Could you check a few things on this model? Use its own coordinates, in mm. A direction names the side the tool comes from. Coordinates: 2 decimals unless noted, no trailing zeros. Order: outer loops, then holes, each group sorted by start corner. A loop starts at its lowest first (then second) coordinate and runs counter-clockwise, first axis right, second up.
```python
from build123d import *

# Parameters (mm, degrees)
SKETCH1_W               = 200
SKETCH1_H               = 180
BOSS_EXTRUDE1_DEPTH     = 90
CUT_EXTRUDE1_DEPTH      = 1
CUT_EXTRUDE1_DEPTH_BACK = 181
CUT_EXTRUDE2_DEPTH      = 201
SHELL1_T                = -1.5
SKETCH6_R               = 2.25
HINGE_HOLES_DEPTH       = 2.5
CUT_EXTRUDE4_DEPTH      = 50


with BuildPart() as part:
    # Sketch1 → Boss-Extrude1 (new body)
    with BuildSketch(Plane(origin=(0, 0, 0), x_dir=(1, 0, 0), z_dir=(0, 1, 0))):
        with Locations((100, 90)):
            Rectangle(SKETCH1_W, SKETCH1_H)
    extrude(amount=BOSS_EXTRUDE1_DEPTH)

    # Sketch4 → Cut-Extrude1 (cut, two sides)
    with BuildSketch(Plane.XY) as cut_extrude1_sk:
        Polygon((0, 85), (30.937469913, 0), (0, 0), align=None)
        Polygon((200, 85), (200, 0), (169.062530087, 0), align=None)
    extrude(amount=CUT_EXTRUDE1_DEPTH, mode=Mode.SUBTRACT)
    extrude(cut_extrude1_sk.sketch, amount=-CUT_EXTRUDE1_DEPTH_BACK, mode=Mode.SUBTRACT)

    # Sketch5 → Cut-Extrude2 (cut, through all)
    with BuildSketch(Plane.ZY):
        Polygon((-180, 85), (-149.062530087, 0), (-180, 0), align=None)
        Polygon((0, 85), (-30.937469913, 0), (0, 0), align=None)
    extrude(amount=-CUT_EXTRUDE2_DEPTH, mode=Mode.SUBTRACT)

    # Shell1
    shell1_openings = [part.faces().sort_by_distance(p)[0] for p in [
        (100, 90, -90),
    ]]
    offset(amount=SHELL1_T, openings=shell1_openings, kind=Kind.INTERSECTION)

    # Sketch6 → Hinge-Holes (cut, through all)
    with BuildSketch(Plane(origin=(0, 1.5, 0), x_dir=(1, 0, 0), z_dir=(0, 1, 0))):
        with Locations((90, 90)):
            Circle(SKETCH6_R)
        with Locations((110, 90)):
            Circle(SKETCH6_R)
    extrude(amount=-HINGE_HOLES_DEPTH, mode=Mode.SUBTRACT)

    # Sketch7 → Cut-Extrude4 (cut)
    with BuildSketch(Plane.XY):
        with BuildLine():
            Line((139.686269666, 85), (60.313730334, 85))
            ThreePointArc((60.313730334, 85), (100, 50), (139.686269666, 85))
        make_face()
        with BuildLine():
            Line((140, 90), (60, 90))
            ThreePointArc((60, 90), (60.078509631, 87.495083498), (60.313730334, 85))
            Line((60.313730334, 85), (139.686269666, 85))
            ThreePointArc((139.686269666, 85), (139.921490369, 87.495083498), (140, 90))
        make_face()
    extrude(amount=-CUT_EXTRUDE4_DEPTH, mode=Mode.SUBTRACT)


solid = part.part
```
Item 1: I need wall thicknesses on line 1 (X direction, y = 0.6, z = -90); line 2 (X direction, y = 0.9, z = -90); line 3 (Y direction, x = 44, z = -147). Which ranges of each line are inside material? Lowest first, please.
Item 2: Suppose I cut it at A-A (y = 47.5). List the corners of the cut face in (x, z) for me, and give its area (3 significant figures).
Item 3: For pin 1 Ø4 at (x, y) = (73, 88) entering from +Z; pin 2 Ø4 at (x, y) = (69.5, 57) entering from -Z; pin 3 Ø1 at (x, y) = (106.5, 39.5) entering from -Z, each with a flat end and sliding along its axis, tell me the tip position at first contact or that it passes through.
Item 4: Suppose I cut it at C-C (z = -129.5). List the corners of the cut face in (x, y) for me, and give its area (3 significant figures).
Item 5: Suppose I cut it at D-D (y = 60). List the corners of the cut face in (x, z) for me, and give its area (3 significant figures).
Item 6: Suppose I cut it at B-B (x = 124). List the corners of the cut face in (y, z) for me.
Item 7: Thinking about a two-plate mould opening in Z: for faces 1 (the face through (112.08, 0.76, -89.14)), 2 (the face through (99, 0, -91)), 3 (the face through (99, 87, -180)), which applies, +Z half, -Z half, draft (parallel to the pull), parting line (faces both ways), or undercut?
Item 8: Which directions (+Z, -Z, +X, -X, +Y, -Y) give clear straight access to the entire face, cutting with the end or side of a thin tool? Please do faces 4 (the face through (200, 87, -89)), 5 (the face through (198.5, 88, -89)).
Geometry results:
1. line 1: x = 30.72 to 87.75, 92.25 to 107.75, 112.25 to 169.28
1. line 2: x = 30.61 to 87.75, 92.25 to 107.75, 112.25 to 169.39
1. line 3: y = 0 to 1.5
2. outline: (13.65, -166.35) - (186.35, -166.35) - (186.35, -13.65) - (13.65, -13.65) - close; hole (15.25, -164.75) - (184.75, -164.75) - (184.75, -15.25) - (15.25, -15.25) - close
2. area: 1,030 mm2
3. pin 1: stops at z = -178.5
3. pin 2: stops at z = -170.54
3. pin 3: stops at z = -163.62
4. outline: (0, 85) - (30.94, 0) - (169.06, 0) - (200, 85) - (200, 90) - (198.5, 90) - (198.5, 85.26) - (168.01, 1.5) - (31.99, 1.5) - (1.5, 85.26) - (1.5, 90) - (0, 90) - close
4. area: 490 mm2
5. outline: (9.1, -170.9) - (190.9, -170.9) - (190.9, -9.1) - (126.46, -9.1) - (126.46, -10.7) - (189.3, -10.7) - (189.3, -169.3) - (10.7, -169.3) - (10.7, -10.7) - (73.54, -10.7) - (73.54, -9.1) - (9.1, -9.1) - close
5. area: 1,000 mm2
6. outline: (0, -149.06) - (85, -180) - (90, -180) - (90, -178.5) - (85.26, -178.5) - (1.5, -148.01) - (1.5, -31.99) - (58, -11.42) - (58, -9.83) - (0, -30.94) - close
7. face 1: undercut
7. face 2: draft
7. face 3: -Z half
8. face 4: +Z, -Z, +X, +Y, -Y
8. face 5: +Y
